Can you work these out from the model? Positions are in its coordinate system, mm. A direction names the side the tool comes from. Round coordinates to 2 decimals unless told otherwise and drop trailing zeros. Loops run counter-clockwise (first coordinate to the right, second up) from the corner with the lowest first, then second, coordinate; pieces in that order, holes last. Notation, with made-up numbers: (53.5, -19) - (103.5, -19) arc R23 ccw to (103.5, 14) - close; hole circle Ø11 at (74.5, 88.5). An arc over 180 degrees is marked (long way). Answer as CSV lines item,"result".
```python
from build123d import *

# Parameters (mm, degrees)
ESQUISSE1_W                                 = 60
ESQUISSE1_H                                 = 74
BOSS_EXTRU_1_DEPTH                          = 3
ESQUISSE2_R                                 = 28
BOSS_EXTRU_2_DEPTH                          = 2
ESQUISSE6_R                                 = 25
ENL_V_MAT_EXTRU_4_DEPTH                     = 0.5
CONG_5_R                                    = 5
CONG_1_R                                    = 1
ESQUISSE7_R                                 = 2.5
ENL_V_MAT_EXTRU_5_DEPTH                     = 48.895720059
FRAISAGE_POUR_VIS_T_TE_FRAIS_E_M31_AT_COUNT = 2
FRAISAGE_POUR_VIS_T_TE_FRAIS_E_M31_AT_PITCH = 64


with BuildPart() as part:
    # Esquisse1 → Boss.-Extru.1 (new body)
    with BuildSketch(Plane.XY):
        Rectangle(ESQUISSE1_W, ESQUISSE1_H)
    extrude(amount=-BOSS_EXTRU_1_DEPTH)

    # Esquisse2 → Boss.-Extru.2 (add)
    with BuildSketch(Plane.XY):
        Circle(ESQUISSE2_R)
    extrude(amount=BOSS_EXTRU_2_DEPTH)

    # Esquisse6 → Enlèv. mat.-Extru.4 (cut)
    with BuildSketch(Plane.XY.offset(2)):
        Circle(ESQUISSE6_R)
    extrude(amount=-ENL_V_MAT_EXTRU_4_DEPTH, mode=Mode.SUBTRACT)

    # Congé 5
    cong_5_edges = [part.edges().sort_by_distance(p)[0] for p in [
        (-30, 37, -1.5),
        (30, 37, -1.5),
        (30, -37, -1.5),
        (-30, -37, -1.5),
    ]]
    fillet(cong_5_edges, radius=CONG_5_R)

    # Congé1
    cong_1_edges = [part.edges().sort_by_distance(p)[0] for p in [
        (-28, 0, 2),
        (0, -37, 0),
        (-30, 0, 0),
        (30, 0, 0),
        (0, 37, 0),
        (-28.535533906, 35.535533906, 0),
        (28.535533906, 35.535533906, 0),
        (-28.535533906, -35.535533906, 0),
        (28.535533906, -35.535533906, 0),
    ]]
    fillet(cong_1_edges, radius=CONG_1_R)

    # Esquisse7 → Enlèv. mat.-Extru.5 (cut, through all)
    with BuildSketch(Plane(origin=(0, 0, -3), x_dir=(-1, 0, 0), z_dir=(0, 0, -1))):
        Circle(ESQUISSE7_R)
    extrude(amount=-ENL_V_MAT_EXTRU_5_DEPTH, mode=Mode.SUBTRACT)

    # Esquisse8 → Fraisage pour vis à tête fraisée M31 (revolve, cut)
    with BuildSketch(Plane(origin=(-9, 32, 0), x_dir=(0, -1, 0), z_dir=(1, 0, 0))):
        Polygon((0, 0), (0, 3), (1.7, 3), (1.7, 1.45), (3.15, 0), align=None)
    fraisage_pour_vis_t_te_frais_e_m31 = revolve(axis=Axis((-9, 32, 6.35), (0, 0, -1)), mode=Mode.SUBTRACT)

    # Fraisage pour vis à tête fraisée M31 at: Fraisage pour vis à tête fraisée M31 ×2
    with Locations(*[(0, -i * FRAISAGE_POUR_VIS_T_TE_FRAIS_E_M31_AT_PITCH, 0) for i in range(1, FRAISAGE_POUR_VIS_T_TE_FRAIS_E_M31_AT_COUNT)]):
        add(fraisage_pour_vis_t_te_frais_e_m31, mode=Mode.SUBTRACT)


solid = part.part
```
Q1. Imagine slicing it at B-B (x = 0). Write out the boundary of the cut face in (y, z).
Checks:
outline,"(-37, -3) - (-2.5, -3) - (-2.5, 1.5) - (-25, 1.5) - (-25, 2) - (-27, 2) arc R1 ccw to (-28, 1) - (-28, 0) - (-36, 0) arc R1 ccw to (-37, -1) - close; (2.5, -3) - (37, -3) - (37, -1) arc R1 ccw to (36, 0) - (28, 0) - (28, 1) arc R1 ccw to (27, 2) - (25, 2) - (25, 1.5) - (2.5, 1.5) - close"
Q2. If I drill on line 1 along Y through (x, z) = (-9, -1.9); line 2 along X through (y, z) = (-32, -2.25); line 3 along Y through (x, z) = (-8, -2), over which ranges is the centre line in solid material (lowest first)? Write a range as [from, to].
Checks:
line 1,"[-37, -33.7], [-30.3, 30.3], [33.7, 37]"
line 2,"[-30, -10.7], [-7.3, 30]"
line 3,"[-37, -33.37], [-30.63, 30.63], [33.37, 37]"
Q3. I'm going to push flat-ended pins straight in: pin 1 Ø3 at (x, y) = (-9, 32) entering from -Z; pin 2 Ø12 at (x, y) = (23.5, 16) entering from +Z; pin 3 Ø1.5 at (y, z) = (-20.5, 1) entering from +X; pin 4 Ø6 at (x, y) = (0, 0) entering from +Z. Where does each tip first touch, or does it pass through?
Checks:
pin 1,"through"
pin 2,"z = 2"
pin 3,"x = 19.85"
pin 4,"z = 1.5"
Q4. We'd pull the mould along Y, two halves only. Please class faces 1 (the flat face through (0, -5, 1.5)), 2 (the flat face through (24, -8, 2)), 3 (the flat face through (0, 37, -2)): pulls with the +Y half, pulls with the -Y half, needs draft (parallel to the pull), parting line crosses it, or undercut.
Checks:
face 1,"undercut"
face 2,"needs draft"
face 3,"pulls with the +Y half"
Q5. Imagine slicing it at A-A (y = 0). Write out the boundary of the cut face in (x, z).
Checks:
outline,"(-30, -3) - (-2.5, -3) - (-2.5, 1.5) - (-25, 1.5) - (-25, 2) - (-27, 2) arc R1 ccw to (-28, 1) - (-28, 0) - (-29, 0) arc R1 ccw to (-30, -1) - close; (2.5, -3) - (30, -3) - (30, -1) arc R1 ccw to (29, 0) - (28, 0) - (28, 1) arc R1 ccw to (27, 2) - (25, 2) - (25, 1.5) - (2.5, 1.5) - close"
Q6. On a 3-axis mill with a long thin cutter (end or side, diameter ignored), from which of +Z, -Z, +X, -X, +Y, -Y can I reach the whole of each face in a straight line? I mean faces 4 (the cylindrical face through (0.54, -2.44, -0.78)), 5 (the cylindrical face through (25.865, -10.724, 0.493)). Say none if no direction works.
Checks:
face 4,"+Z, -Z"
face 5,"+Z"
